Input: part model. Units: mm. Frame: model coordinates. Face numbers are marked on the shaded views. Coordinates: 2 decimals unless noted, no trailing zeros. Loops run counter-clockwise (first coordinate to the right, second up) from the corner with the lowest first, then second, coordinate; pieces in that order, holes last. Notation, with made-up numbers: (28.5, 28.5) -> (58.5, 28.5) arc R21 cw to (58.5, 45.5) -> close; hole circle Ø9 at (42.5, 4). An arc over 180 degrees is marked (long way). Answer as a JSON object with one key per item and string values.
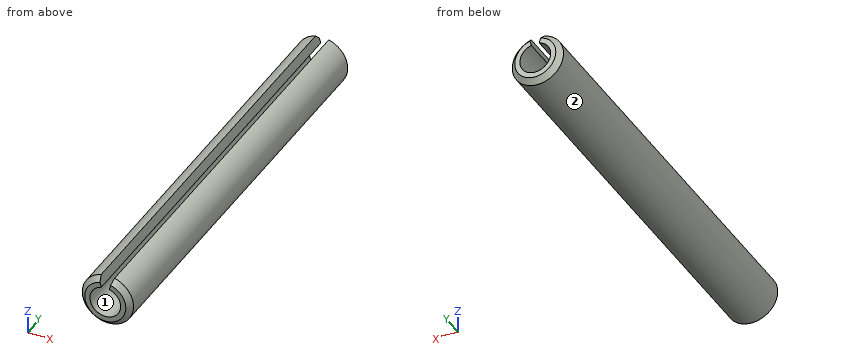
from build123d import *

# Parameters (mm, degrees)
F0_R     = 1.5
F1_DEPTH = 25
F2_T     = -0.6
F3_SIZE  = 0.3
F4_SIZE  = 0.3
F6_DEPTH = 25.001


with BuildPart() as f1:
    # F0 (on Front) → F1 (new body)
    with BuildSketch(Plane.XZ):
        Circle(F0_R)
    extrude(amount=F1_DEPTH)

    # F2
    f2_openings = [f1.faces().sort_by_distance(p)[0] for p in [
        (0, -25, 0),
        (0, 0, 0),
    ]]
    offset(amount=F2_T, openings=f2_openings)

    # F3
    f3_edges = [f1.edges().sort_by_distance(p)[0] for p in [
        (-1.5, -25, 0),
    ]]
    chamfer(f3_edges, length=F3_SIZE)

    # F4
    f4_edges = [f1.edges().sort_by_distance(p)[0] for p in [
        (-1.5, 0, 0),
    ]]
    chamfer(f4_edges, length=F4_SIZE)

    # F5 (on face) → F6 (cut, through all)
    with BuildSketch(Plane.XZ.offset(25)):
        Polygon((-0.489606, 1.827236), (0, 0), (0.489606, 1.827236), align=None)
    extrude(amount=-F6_DEPTH, mode=Mode.SUBTRACT)


solid = f1.part
1. Line query: line 1 along X through (y, z) = (-13.25, 0); line 2 along X through (y, z) = (-8, 0.3); line 3 along Z through (x, y) = (-0.75, -20.5). Output: solid intervals per line, ascending.
Reply:
{"line 1": "x = -1.5 to -0.9, 0.9 to 1.5", "line 2": "x = -1.47 to -0.85, 0.85 to 1.47", "line 3": "z = -1.3 to -0.5, 0.5 to 1.3"}
2. Section query C-C (y = -2.75). Return loops of the section in (x, z).
Reply:
{"outline": "(-0.39, 1.45) arc R1.5 ccw (long way) to (0.39, 1.45) -> (0.23, 0.87) arc R0.9 cw (long way) to (-0.23, 0.87) -> close"}
3. Mould query, pull axis X, two halves, no side actions, for the marked faces 1 and 2. Classes: pulls with the +X half, pulls with the -X half, needs draft (parallel to the pull), parting line crosses it, or undercut.
Reply:
{"face 1": "undercut", "face 2": "parting line crosses it"}
4. Section query A-A (z = 0). Return loops of the section in (x, y), plus the area to 3 significant figures.
Reply:
{"outline": "(-1.5, -24.7) -> (-1.2, -25) -> (-0.9, -25) -> (-0.9, 0) -> (-1.2, 0) -> (-1.5, -0.3) -> close; (0.9, -25) -> (1.2, -25) -> (1.5, -24.7) -> (1.5, -0.3) -> (1.2, 0) -> (0.9, 0) -> close", "area": "29.8 mm2"}
5. Pin query (flat end, axial travel): P1, Ø1, axis at x = -1, y = -12.5, coming from the -Z side; P2, Ø1.4, axis at x = 0, z = 0, coming from the -Y side. Return the tip coordinate at first contact, or that it passes through.
Reply:
{"P1": "stops at z = -1.41", "P2": "passes through"}
6. Section query B-B (x = 0). Return loops of the section in (y, z).
Reply:
{"outline": "(-25, -1.2) -> (-24.7, -1.5) -> (-0.3, -1.5) -> (0, -1.2) -> (0, -0.9) -> (-25, -0.9) -> close"}
